The listing builds one solid part. Answer for the finished solid, in the listing's coordinates (mm). A direction names the side the tool comes from. Round coordinates to 2 decimals unless told otherwise and drop trailing zeros. Loops run counter-clockwise (first coordinate to the right, second up) from the corner with the lowest first, then second, coordinate; pieces in that order, holes last. Notation, with made-up numbers: (-1.5, 31.25) -> (6.5, 31.25) arc R11 cw to (6.5, 51.25) -> close; hole circle Ø3 at (36.5, 34). An arc over 180 degrees is marked (long way). One line per question, with ' | ' between items.
from build123d import *

# Parameters (mm, degrees)
F1_R         = 15.4658150948
F3_DEPTH     = 25.4
F0_W         = 91.367084533
F0_H         = 30.8810528368
F4_DEPTH     = 25.4
F2_R         = 15.313452945
F5_DEPTH     = 25.4
F6_R         = 3.9725855112
F7_DEPTH     = 25.4
F8_R         = 4.5697295071
F9_DEPTH     = 26.67
F10_R        = 3.9038322972
F11_DEPTH    = 30.988
F12_W        = 45.4270541668
F12_H        = 13.8839902356
F13_DEPTH    = 29.718
F15_R        = 10.7036365959
F16_DEPTH    = 25.4
F17_R        = 10.3585042146
F18_DEPTH    = 46.736
F14_R        = 2.4093664871
F19_DEPTH    = 44.196
F20_R        = 5.08
F21_T1_DEPTH = 39.2839902356


# Not quite as in the source:
# - a fillet or chamfer that OpenCascade refuses, or shapes differently, is made with other operations: its cross-section is extruded or revolved along the edge and cut away or added


with BuildPart() as f3:
    # F1 (on Top) → F3 (new body)
    with BuildSketch(Plane.XY):
        with Locations((-45.811150223, 0)):
            Circle(F1_R)
    extrude(amount=F3_DEPTH)

    # F0 (on Top) → F4 (join)
    with BuildSketch(Plane.XY):
        with Locations((0.1276079565, -0.2552149817)):
            Rectangle(F0_W, F0_H)
    extrude(amount=F4_DEPTH)

    # F2 (on Top) → F5 (join)
    with BuildSketch(Plane.XY):
        with Locations((45.55593431, 0)):
            Circle(F2_R)
    extrude(amount=F5_DEPTH)

    # F6 (on Top) → F7 (cut)
    with BuildSketch(Plane.XY):
        with Locations((-53.0294403434, 0)):
            Circle(F6_R)
    extrude(amount=-F7_DEPTH, mode=Mode.SUBTRACT)

    # F8 (on Top) → F9 (cut)
    with BuildSketch(Plane.XY):
        with Locations((-52.3779653013, 0)):
            Circle(F8_R)
    extrude(amount=F9_DEPTH, mode=Mode.SUBTRACT)

    # F10 (on Top) → F11 (cut)
    with BuildSketch(Plane.XY):
        with Locations((52.7567230165, 0)):
            Circle(F10_R)
    extrude(amount=F11_DEPTH, mode=Mode.SUBTRACT)

    # F12 (on Top) → F13 (join)
    with BuildSketch(Plane.XY):
        with Locations((0.0732727349, -0.3520357423)):
            Rectangle(F12_W, F12_H)
    extrude(amount=-F13_DEPTH)

    # F15 (on Front) → F16 (cut)
    with BuildSketch(Plane.XZ):
        with Locations((0, -29.8675838858)):
            Circle(F15_R)
    extrude(amount=-F16_DEPTH, mode=Mode.SUBTRACT)

    # F17 (on Front) → F18 (cut)
    with BuildSketch(Plane.XZ):
        with Locations((0, -27.270803228)):
            Circle(F17_R)
    extrude(amount=F18_DEPTH, mode=Mode.SUBTRACT)

    # F14 (on Right) → F19 (cut)
    with BuildSketch(Plane.YZ):
        with Locations((0, -25.1646973193)):
            Circle(F14_R)
    extrude(amount=F19_DEPTH, mode=Mode.SUBTRACT)

    # F20
    f20_edges = [f3.edges().sort_by_distance(p)[0] for p in [
        (-22.640254, -0.352036, -29.718),
    ]]
    fillet(f20_edges, radius=F20_R)

    # F21: fillet of radius 5.08 on 1 edges, made by hand

    # F21_s2 → F21_t1 (cut)
    with BuildSketch(Plane.XZ.offset(-19.2899593756)):
        with BuildLine():
            ThreePointArc((22.7867998183, -24.638), (21.2989022667, -28.2301024484), (17.7067998183, -29.718))
            Line((17.7067998183, -29.718), (22.7867998183, -29.718))
            Line((22.7867998183, -29.718), (22.7867998183, -24.638))
        make_face()
    extrude(amount=F21_T1_DEPTH, mode=Mode.SUBTRACT)


solid = f3.part
Q1. A cutting plane is placed at A-A on z = 13. Give the vertices of the cut face in (x, y).
Numbers:
outline: (-45.56, -15.7) -> (45.81, -15.7) -> (45.81, -15.31) arc R15.31 ccw (long way) to (43.58, 15.19) -> (-42.88, 15.19) arc R15.47 ccw (long way) to (-45.56, -15.46) -> close; hole circle Ø9.14 at (-52.38, 0); hole circle Ø7.81 at (52.76, 0)
Q2. Find the intervals of material crossed by line 1 (X direction, y = 0, z = 5.5); line 2 (Z direction, x = 0, y = -2.75); line 3 (Z direction, x = 17, y = 0), in increasing order. Write a range as from..to.
Numbers:
line 1: -61.28..-56.95, -47.81..48.85, 56.66..60.87 | line 2: -16.91..25.4 | line 3: -29.72..-27.57, -22.76..25.4
Q3. A cutting plane is placed at C-C on z = -11. Give the vertices of the cut face in (x, y).
Numbers:
outline: (-22.64, -7.29) -> (22.79, -7.29) -> (22.79, 6.59) -> (-22.64, 6.59) -> close
Q4. A cutting plane is placed at D-D on x = -13. Give the vertices of the cut face in (y, z).
Numbers:
outline: (-15.7, 0) -> (-7.29, 0) -> (-7.29, -29.72) -> (6.59, -29.72) -> (6.59, 0) -> (15.19, 0) -> (15.19, 25.4) -> (-15.7, 25.4) -> close
Q5. For a pull along Y with two mould halves and no side action, classify faces 1 (the face through (14, 0, -29.718)), 2 (the face through (-48.02, 1.37, 12.52)), 3 (the face through (15.289, -0.314, -22.776)), 4 (the face through (0, -7.294, -11)) as pulls with the +Y half, pulls with the -Y half, needs draft (parallel to the pull), parting line crosses it, or undercut.
Numbers:
face 1: needs draft | face 2: undercut | face 3: undercut | face 4: pulls with the -Y half
Q6. A cutting plane is placed at B-B on x = 0. Give the vertices of the cut face in (y, z).
Numbers:
outline: (-15.7, 0) -> (-7.29, 0) -> (-7.29, -16.91) -> (0, -16.91) -> (0, -19.16) -> (6.59, -19.16) -> (6.59, 0) -> (15.19, 0) -> (15.19, 25.4) -> (-15.7, 25.4) -> close
Q7. For faces 5 (the face through (0, 6.59, -11)), 6 (the face through (-22.64, 0, -12)), 7 (the face through (0, 15.185, 13)), 8 (the face through (0.233, 3.249, -19.166)), determine the directions among +Z, -Z, +X, -X, +Y, -Y from which every point of the face is accessible in a straight line to the end or side of a thin tool.
Numbers:
face 5: -Z, +X, -X, +Y | face 6: -Z, -X, +Y, -Y | face 7: +Z, -Z, +Y | face 8: -Z, +Y
Q8. Given pin 1 Ø20.5 at (x, z) = (6, 13.5) entering from +Y; pin 2 Ø12 at (y, z) = (10.5, -23.5) entering from -X; pin 3 Ø1.5 at (x, z) = (0.5, -3) entering from -Y, each flat-ended and moving along its own axis, determine where each tip first touches the part or whether it passes through.
Numbers:
pin 1: y = 15.19 | pin 2: x = -22.64 | pin 3: y = -7.29
